Read the model definition and answer for the solid it produces. Units are mm, in the model's axes. Coordinates: 2 decimals unless noted, no trailing zeros. Write each loop counter-clockwise with the first axis right and the second up, starting at its lowest first coordinate (ties: lowest second). Pieces come first, ordered by that corner, then holes. Notation, with made-up numbers: (59, 14) -> (84, 14) arc R33 ccw to (84, 48) -> close; hole circle Ø11 at (-19.5, 49.5). An arc over 180 degrees is marked (long way). One line per item, written item: value. Start each with the question number.
1. Consider line 1 along Y through (x, z) = (-47, 0); line 2 along Z through (x, y) = (-63, -8); line 3 along X through (y, z) = (168.5, 110). Determine where each line is inside the solid, lowest interval first.
2. Find section A-A, the plane z = 0. Write down the section's boundary in (x, y), and give its area (3 significant figures).
3. For a pull along Y with two mould halves and no side action, classify faces 1 (the cylindrical face through (-59.132, -141.622, 144.903)), 2 (the cylindrical face through (1.12, 244.35, 56.2)), 3 (the cylindrical face through (58.546, -141.622, 144.903)), 4 (the flat face through (-79.773, -202, -40)) as pulls with the +Y half, pulls with the -Y half, needs draft (parallel to the pull), parting line crosses it, or undercut.
4. Given P1, Ø5, axis at x = -1, z = -100.5, coming from the +Y side; P2, Ø1.5, axis at x = 50.5, z = -199, coming from the -Y side; P3, Ø4, axis at y = 183, z = 177.5, coming from the -X side; P4, Ø6, axis at x = -42, y = -51.5, coming from the +Z side, each flat-ended and moving along its own axis, determine where each tip first touches the part or whether it passes through.
5. Find section B-B, the plane x = -48. Write down the section's boundary in (y, z), and give its area (3 significant figures).
6. Find section C-C, the plane x = 15. Write down the section's boundary in (y, z), and give its area (3 significant figures).
```python
from build123d import *

# Parameters (mm, degrees)
SCALE2_SCALE = 6
SCALE3_SCALE = 3.323882225


with BuildPart() as part:
    # Sketch1 → Revolve1 (revolve)
    with BuildSketch(Plane.XY, mode=Mode.PRIVATE) as revolve1_sk:
        with BuildLine():
            Line((0, 4.25), (4, 4.25))
            Line((4, 4.25), (4, 1.108))
            Line((4, 1.108), (1.900614637, 1.108))
            ThreePointArc((1.900614637, 1.108), (0, 2.2), (-1.900614637, 1.108))
            Line((-1.900614637, 1.108), (-4, 1.108))
            Line((-4, 1.108), (-4, 4.25))
            Line((-4, 4.25), (0, 4.25))
        make_face()
    revolve(revolve1_sk.sketch.rotate(Axis((4, -8.75, 0), (-1, 0, 0)), 90), axis=Axis((4, -8.75, 0), (-1, 0, 0)))


with BuildPart() as part_1:
    # Scale2: scaled about (0, -8.75, 0)
    add(part.part.scale(SCALE2_SCALE).moved(Location((0, 43.75, 0))))


with BuildPart() as part_2:
    # Scale3: scaled about (0, -8.75, 0)
    add(part_1.part.scale(SCALE3_SCALE).moved(Location((0, 20.333969466, 0))))


solid = part_2.part
```
Answer block:
1. line 1: y = -268.01 to -205.35, 187.85 to 250.51
1. line 2: z = -259.26 to -196.6, 196.6 to 259.26
1. line 3: x = -79.77 to -27.6, 27.6 to 79.77
2. outline: (-79.77, -268.01) -> (79.77, -268.01) -> (79.77, -205.35) -> (37.9, -205.35) arc R43.88 cw to (-37.9, -205.35) -> (-79.77, -205.35) -> close; (-79.77, 187.85) -> (-37.9, 187.85) arc R43.88 cw to (37.9, 187.85) -> (79.77, 187.85) -> (79.77, 250.51) -> (-79.77, 250.51) -> close
2. area: 17,700 mm2
3. face 1: undercut
3. face 2: parting line crosses it
3. face 3: undercut
3. face 4: needs draft
4. P1: stops at y = 231.28
4. P2: stops at y = -175.83
4. P3: passes through
4. P4: stops at z = 256.2
5. outline: circle Ø518.53 at (-8.75, 0); hole circle Ø393.2 at (-8.75, 0)
5. area: 89,700 mm2
6. outline: circle Ø518.53 at (-8.75, 0); hole circle Ø431.47 at (-8.75, 0)
6. area: 65,000 mm2
